Geometry check sheet. Reference: the model listing, model coordinates, mm. Face numbers are marked on the shaded views. A direction names the side the tool comes from. Coordinates: 2 decimals unless noted, no trailing zeros. Loops run counter-clockwise (first coordinate to the right, second up) from the corner with the lowest first, then second, coordinate; pieces in that order, holes last. Notation, with made-up numbers: (30, -5.75) -> (57, -5.75) arc R34 ccw to (57, 29.25) -> close; hole circle Ø8 at (89.25, 84). An arc over 180 degrees is marked (long way). Answer as a JSON object with one key per item and string values.
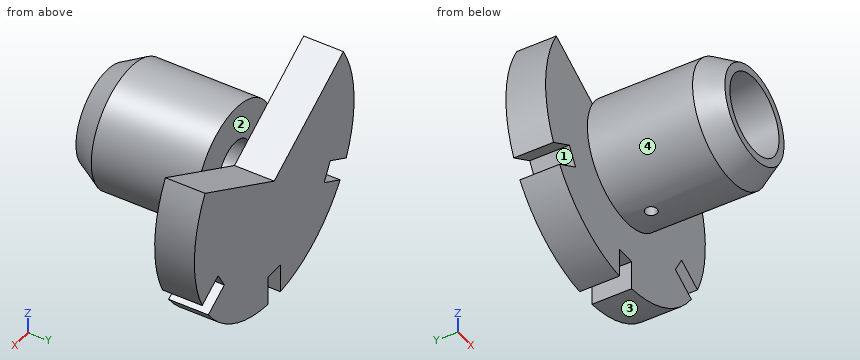
from build123d import *

# Parameters (mm, degrees)
ESTRUSIONE_ESTRUSIONE1_DEPTH = 20
SCHIZZO2_R                   = 31
ESTRUSIONE_ESTRUSIONE2_DEPTH = 65
SCHIZZO3_R                   = 20
TAGLIO_ESTRUSIONE1_DEPTH     = 26
FORO_25_0_25_1_D             = 25
FORO_25_0_25_1_DEPTH         = 39
FORO_6_0_6_1_REACH           = 113.724
FORO_6_0_6_1_BORE_R          = 3
SMUSSO1_SIZE                 = 12
SMUSSO1_SIZE2                = 6.92820323


with BuildPart() as part:
    # Schizzo1 → Estrusione-Estrusione1 (new body)
    with BuildSketch(Plane(origin=(0, 0, 0), x_dir=(1, 0, 0), z_dir=(0, 1, 0))):
        with BuildLine():
            Line((0, 0), (-56.291651246, -32.5))
            ThreePointArc((-56.291651246, -32.5), (-64.9518339, -2.501853916), (-58.624860802, 28.073576473))
            Line((-58.624860802, 28.073576473), (-45.634479745, 20.573576473))
            Line((-45.634479745, 20.573576473), (-40.634479745, 29.233830511))
            Line((-40.634479745, 29.233830511), (-53.624860802, 36.733830511))
            ThreePointArc((-53.624860802, 36.733830511), (-32.5, 56.291651246), (-5, 64.807406984))
            Line((-5, 64.807406984), (-5, 49.807406984))
            Line((-5, 49.807406984), (5, 49.807406984))
            Line((5, 49.807406984), (5, 64.807406984))
            ThreePointArc((5, 64.807406984), (32.5, 56.291651246), (53.624860802, 36.733830511))
            Line((53.624860802, 36.733830511), (40.634479745, 29.233830511))
            Line((40.634479745, 29.233830511), (45.634479745, 20.573576473))
            Line((45.634479745, 20.573576473), (58.624860802, 28.073576473))
            ThreePointArc((58.624860802, 28.073576473), (64.9518339, -2.501853916), (56.291651246, -32.5))
            Line((56.291651246, -32.5), (0, 0))
        make_face()
    extrude(amount=ESTRUSIONE_ESTRUSIONE1_DEPTH)

    # Schizzo2 → Estrusione-Estrusione2 (add)
    with BuildSketch(Plane.XZ):
        with Locations(Location((0, 0, 0), (0, 0, 150))):
            Circle(SCHIZZO2_R)
    extrude(amount=ESTRUSIONE_ESTRUSIONE2_DEPTH)

    # Schizzo3 → Taglio-Estrusione1 (cut)
    with BuildSketch(Plane.XZ.offset(65)):
        with Locations(Location((0, 0, 0), (0, 0, 270))):
            Circle(SCHIZZO3_R)
    extrude(amount=-TAGLIO_ESTRUSIONE1_DEPTH, mode=Mode.SUBTRACT)

    # Foro Ø25.0 (25)-1
    with Locations(Plane(origin=(0, -39, 0), x_dir=(-1, 0, 0), z_dir=(0, -1, 0))):
        with Locations((0, 0)):
            Hole(FORO_25_0_25_1_D / 2, depth=FORO_25_0_25_1_DEPTH)

    # Foro Ø6.0 (6)-1 bore → Foro Ø6.0 (6)-1 (cut, up to next)
    with BuildSketch(Plane(origin=(0, 0, -31), x_dir=(-1, 0, 0), z_dir=(0, 0, -1)), mode=Mode.PRIVATE) as foro_6_0_6_1_sk1:
        with Locations((0, -13)):
            Circle(FORO_6_0_6_1_BORE_R)
    foro_6_0_6_1_tool1 = extrude(foro_6_0_6_1_sk1.sketch, amount=-FORO_6_0_6_1_REACH, mode=Mode.PRIVATE) & part.part
    add(foro_6_0_6_1_tool1.solids().sort_by_distance((0, -13, -31))[0], mode=Mode.SUBTRACT)

    # Smusso1
    smusso1_edges = [part.edges().sort_by_distance(p)[0] for p in [
        (26.846787517, -65, -15.5),
    ]]
    smusso1_side = [part.faces().sort_by_distance(p)[0] for p in [
        (26.846787517, -32.5, -15.5),
    ]]
    chamfer(smusso1_edges, length=SMUSSO1_SIZE, length2=SMUSSO1_SIZE2, reference=smusso1_side[0])


solid = part.part
1. Section check B-B, the plane x = 44. Record the boundary of the cut face in (y, z), then the cut area to 3 significant figures.
Evaluation:
{"outline": "(0, -47.84) -> (20, -47.84) -> (20, -31.18) -> (0, -31.18) -> close; (0, -23.4) -> (20, -23.4) -> (20, 25.4) -> (0, 25.4) -> close", "area": "1,310 mm^2"}
2. Section check C-C, the plane y = -3.5. Record the boundary of the cut face in (x, z), then the cut area to 3 significant figures.
Evaluation:
{"outline": "circle Ø62 at (0, 0); hole circle Ø25 at (0, 0)", "area": "2,530 mm^2"}
3. Thickness scan on probe 1 along X at (y, z) = (-45.5, 0); probe 2 along X at (y, z) = (-16, -0.5); probe 3 along Y at (x, z) = (0, -18.5). Record the ranges inside material, lowest first. Write a range as from..to.
Evaluation:
{"probe 1": "x = -31..-20, 20..31", "probe 2": "x = -31..-12.49, 12.49..31", "probe 3": "y = -39..-16, -10..20"}
4. Tool access check on the marked faces 1, 2, 3 and 4. Record the directions out of +Z, -Z, +X, -X, +Y, -Y that give a thin tool (end or side, any length) a straight path to the whole face; none if there is none.
Evaluation:
{"face 1": "+Y, -Y", "face 2": "+Z, +Y", "face 3": "-Z, +X, +Y, -Y", "face 4": "-Y"}
5. Section check D-D, the plane z = -42. Record the boundary of the cut face in (x, y).
Evaluation:
{"outline": "(-49.61, 0) -> (49.61, 0) -> (49.61, 20) -> (-49.61, 20) -> close"}
6. Section check A-A, the plane z = -54. Record the boundary of the cut face in (x, y).
Evaluation:
{"outline": "(-36.18, 0) -> (-5, 0) -> (-5, 20) -> (-36.18, 20) -> close; (5, 0) -> (36.18, 0) -> (36.18, 20) -> (5, 20) -> close"}
7. Depth check by flat-ended pin: P1, Ø3, axis at x = -1, y = 6.5, coming from the -Z side; P2, Ø5, axis at x = 2.5, y = -5.5, coming from the -Z side; P3, Ø12, axis at x = -39.5, z = -47, coming from the -Y side; P4, Ø12, axis at x = 15, z = -0.5, coming from the -Y side. Enter the tip coordinate at first touch or a pass-through.
Evaluation:
{"P1": "stops at z = -49.81", "P2": "stops at z = -31", "P3": "stops at y = 0", "P4": "stops at y = -65"}
